Geometry: final body of the model. Coordinates: model frame, mm. A direction names the side the tool comes from. Round coordinates to 2 decimals unless told otherwise and drop trailing zeros. Write each loop counter-clockwise with the first axis right and the second up, starting at its lowest first coordinate (ties: lowest second). Pieces come first, ordered by that corner, then holes. Notation, with made-up numbers: (29, 13) - (34, 13) arc R26 ccw to (34, 27) - close; hole circle Ø3 at (42, 5). An arc over 180 degrees is marked (long way). Use a Markdown table: item, result. Add a question column.
```python
from build123d import *

# Parameters (mm, degrees)
PARED_START                    = -27.5
SK_PARED_W                     = 50
SK_PARED_H                     = 64
PARED_DEPTH                    = 6
CABEZA_START                   = -27.5
SK_CABEZA_R                    = 25
CABEZA_DEPTH                   = 6
ASIENTO_1MM_START              = -21.5
SK_ASIENTO_1MM_R               = 24
SK_ASIENTO_1MM_R_2             = 15
ASIENTO_1MM_DEPTH              = 1
PASO_CENTRAL_START             = -27.5
SK_PASO_CENTRAL_R              = 8
PASO_CENTRAL_DEPTH             = 7
PASANTES_M2_5_ESTATOR_J5_START = -27.5
SK_PASANTES_M2_5_ESTATOR_J5_R  = 1.45
PASANTES_M2_5_ESTATOR_J5_DEPTH = 7
CAJAS_M2_5_J5_START            = -27.5
SK_CAJAS_M2_5_J5_R             = 2.75
CAJAS_M2_5_J5_DEPTH            = 2.5
PASANTES_M4_ANGULOS_START      = -27.5
SK_PASANTES_M4_ANGULOS_R       = 2.25
PASANTES_M4_ANGULOS_DEPTH      = 6


with BuildPart() as part:
    # Sk_Pared → Pared (new body)
    with BuildSketch(Plane(origin=(0, 0, 0), x_dir=(1, 0, 0), z_dir=(0, 1, 0)).offset(PARED_START)):
        with Locations((0, -458)):
            Rectangle(SK_PARED_W, SK_PARED_H)
    extrude(amount=PARED_DEPTH)

    # Sk_Cabeza → Cabeza (add)
    with BuildSketch(Plane(origin=(0, 0, 0), x_dir=(1, 0, 0), z_dir=(0, 1, 0)).offset(CABEZA_START)):
        with Locations((0, -490)):
            Circle(SK_CABEZA_R)
    extrude(amount=CABEZA_DEPTH)

    # Sk_Asiento_1mm → Asiento_1mm (add)
    with BuildSketch(Plane(origin=(0, 0, 0), x_dir=(1, 0, 0), z_dir=(0, 1, 0)).offset(ASIENTO_1MM_START)):
        with Locations(Location((0, -490, 0), (0, 0, 270))):
            Circle(SK_ASIENTO_1MM_R)
        with Locations(Location((0, -490, 0), (0, 0, 270))):
            Circle(SK_ASIENTO_1MM_R_2, mode=Mode.SUBTRACT)
    extrude(amount=ASIENTO_1MM_DEPTH)

    # Sk_Paso_central → Paso_central (cut)
    with BuildSketch(Plane(origin=(0, 0, 0), x_dir=(1, 0, 0), z_dir=(0, 1, 0)).offset(PASO_CENTRAL_START)):
        with Locations(Location((0, -490, 0), (0, 0, 90))):
            Circle(SK_PASO_CENTRAL_R)
    extrude(amount=PASO_CENTRAL_DEPTH, mode=Mode.SUBTRACT)

    # Sk_Pasantes_M2-5_estator_J5 → Pasantes_M2-5_estator_J5 (cut)
    with BuildSketch(Plane(origin=(0, 0, 0), x_dir=(1, 0, 0), z_dir=(0, 1, 0)).offset(PASANTES_M2_5_ESTATOR_J5_START)):
        with Locations(Location((20.5, -490, 0), (0, 0, 270))):
            Circle(SK_PASANTES_M2_5_ESTATOR_J5_R)
        with Locations(Location((10.25, -507.753520778, 0), (0, 0, 270))):
            Circle(SK_PASANTES_M2_5_ESTATOR_J5_R)
        with Locations(Location((-10.25, -507.753520778, 0), (0, 0, 270))):
            Circle(SK_PASANTES_M2_5_ESTATOR_J5_R)
        with Locations(Location((-20.5, -490, 0), (0, 0, 270))):
            Circle(SK_PASANTES_M2_5_ESTATOR_J5_R)
        with Locations(Location((-10.25, -472.246479222, 0), (0, 0, 270))):
            Circle(SK_PASANTES_M2_5_ESTATOR_J5_R)
        with Locations(Location((10.25, -472.246479222, 0), (0, 0, 270))):
            Circle(SK_PASANTES_M2_5_ESTATOR_J5_R)
    extrude(amount=PASANTES_M2_5_ESTATOR_J5_DEPTH, mode=Mode.SUBTRACT)

    # Sk_Cajas_M2-5_J5 → Cajas_M2-5_J5 (cut)
    with BuildSketch(Plane(origin=(0, 0, 0), x_dir=(1, 0, 0), z_dir=(0, 1, 0)).offset(CAJAS_M2_5_J5_START)):
        with Locations(Location((10.25, -507.753520778, 0), (0, 0, 270))):
            Circle(SK_CAJAS_M2_5_J5_R)
        with Locations(Location((-10.25, -507.753520778, 0), (0, 0, 270))):
            Circle(SK_CAJAS_M2_5_J5_R)
        with Locations(Location((-10.25, -472.246479222, 0), (0, 0, 270))):
            Circle(SK_CAJAS_M2_5_J5_R)
        with Locations(Location((10.25, -472.246479222, 0), (0, 0, 270))):
            Circle(SK_CAJAS_M2_5_J5_R)
    extrude(amount=CAJAS_M2_5_J5_DEPTH, mode=Mode.SUBTRACT)

    # Sk_Pasantes_M4_angulos → Pasantes_M4_angulos (cut)
    with BuildSketch(Plane(origin=(0, 0, 0), x_dir=(1, 0, 0), z_dir=(0, 1, 0)).offset(PASANTES_M4_ANGULOS_START)):
        with Locations(Location((-20, -437.11, 0), (0, 0, 270))):
            Circle(SK_PASANTES_M4_ANGULOS_R)
        with Locations(Location((20, -437.11, 0), (0, 0, 270))):
            Circle(SK_PASANTES_M4_ANGULOS_R)
    extrude(amount=PASANTES_M4_ANGULOS_DEPTH, mode=Mode.SUBTRACT)


solid = part.part
```
1) Pin query (flat end, axial travel): P1, Ø18.5, axis at x = 0, z = 490, coming from the +Y side; P2, Ø1, axis at x = 11.5, y = -23.5, coming from the +Z side; P3, Ø1.6, axis at x = 10.5, z = 506.5, coming from the -Y side. Return the tip coordinate at first contact, or that it passes through.
2) Section A-A, the plane y = -26.5. State how many separate pieces and enclosed holes the cut face has, then the cut area to 3 significant figures.
3) Draft query along X for faces 1 (the flat face through (9.1, -25, 473.4)), 2 (the flat face through (0, -25, 426)), 3 (the cylindrical face through (10.371, -26.268, 505.006)), 4 (the cylindrical face through (-0.55, -24.542, 514.994)). Return one class per face: released by +X, released by -X, zero draft, split by the parting line, or undercut.
4) Set-up query: faces 5 (the cylindrical face through (20.099, -24.542, 434.862)), 6 (the flat face through (6, -21.5, 496)), 7 (the cylindrical face through (10.4, -26.3, 469.5)). Return all of +Z, -Z, +X, -X, +Y, -Y with unobstructed straight access to the full face (end or side cutting, diameter ignored); none if empty.
5) Section C-C, the plane z = 437. Return the cut outline in (x, y).
6) Material intervals for L1, parallel to X at y = -21.2, z = 490; L2, parallel to X at y = -23.5, z = 490; L3, parallel to X at y = -23.8, z = 437.11, sorted ascending. Write a range as from..to.
7) Section B-B, the plane x = 10.25. Return the cut outline in (y, z).
Output values:
| question | item | result |
|---|---|---|
| 1 | P1 | stops at y = -21.5 |
| 1 | P2 | stops at z = 512.45 |
| 1 | P3 | stops at y = -25 |
| 2 | separate pieces | 1 |
| 2 | enclosed holes | 9 |
| 2 | area | 3,840 mm^2 |
| 3 | face 1 | undercut |
| 3 | face 2 | zero draft |
| 3 | face 3 | undercut |
| 3 | face 4 | split by the parting line |
| 4 | face 5 | +Y, -Y |
| 4 | face 6 | +Y |
| 4 | face 7 | -Y |
| 5 | outline | (-25, -27.5) - (-22.25, -27.5) - (-22.25, -21.5) - (-25, -21.5) - close; (-17.75, -27.5) - (17.75, -27.5) - (17.75, -21.5) - (-17.75, -21.5) - close; (22.25, -27.5) - (25, -27.5) - (25, -21.5) - (22.25, -21.5) - close |
| 6 | L1 | x = -24..-21.95, -19.05..-15, 15..19.05, 21.95..24 |
| 6 | L2 | x = -25..-21.95, -19.05..-8, 8..19.05, 21.95..25 |
| 6 | L3 | x = -25..-22.25, -17.75..17.75, 22.25..25 |
| 7 | outline | (-27.5, 426) - (-21.5, 426) - (-21.5, 468.3) - (-20.5, 468.3) - (-20.5, 470.8) - (-25, 470.8) - (-25, 469.5) - (-27.5, 469.5) - close; (-27.5, 475) - (-25, 475) - (-25, 473.7) - (-20.5, 473.7) - (-20.5, 479.05) - (-21.5, 479.05) - (-21.5, 500.95) - (-20.5, 500.95) - (-20.5, 506.3) - (-25, 506.3) - (-25, 505) - (-27.5, 505) - close; (-27.5, 510.5) - (-25, 510.5) - (-25, 509.2) - (-20.5, 509.2) - (-20.5, 511.7) - (-21.5, 511.7) - (-21.5, 512.8) - (-27.5, 512.8) - close |
